from build123d import *

# Parameters (mm, degrees)
SKETCH1_W           = 18.5
SKETCH1_H           = 6
SKETCH1_R           = 1.6
BOSS_EXTRUDE1_DEPTH = 3
SKETCH2_W           = 3
SKETCH2_H           = 6
BOSS_EXTRUDE2_DEPTH = 15.5
SKETCH3_R           = 1.6
CUT_EXTRUDE1_DEPTH  = 25.320773014
BOSS_EXTRUDE3_DEPTH = 6


with BuildPart() as part:
    # Sketch1 → Boss-Extrude1 (new body)
    with BuildSketch(Plane(origin=(0, 0, 0), x_dir=(1, 0, 0), z_dir=(0, 1, 0))):
        Rectangle(SKETCH1_W, SKETCH1_H)
        with Locations(Location((-6.25, 0, 0), (0, 0, 270))):
            Circle(SKETCH1_R, mode=Mode.SUBTRACT)
        with Locations(Location((1.75, 0, 0), (0, 0, 270))):
            Circle(SKETCH1_R, mode=Mode.SUBTRACT)
    extrude(amount=BOSS_EXTRUDE1_DEPTH)

    # Sketch2 → Boss-Extrude2 (add)
    with BuildSketch(Plane(origin=(0, 3, 0), x_dir=(1, 0, 0), z_dir=(0, 1, 0))):
        with Locations((7.75, 0)):
            Rectangle(SKETCH2_W, SKETCH2_H)
    extrude(amount=BOSS_EXTRUDE2_DEPTH)

    # Sketch3 → Cut-Extrude1 (cut, through all)
    with BuildSketch(Plane.ZY.offset(-6.25)):
        with Locations((0, 7)):
            Circle(SKETCH3_R)
        with Locations((0, 15)):
            Circle(SKETCH3_R)
    extrude(amount=-CUT_EXTRUDE1_DEPTH, mode=Mode.SUBTRACT)

    # Sketch5 → Boss-Extrude3 (add)
    with BuildSketch(Plane(origin=(6.25, 3, 3), x_dir=(1, 0, 0), z_dir=(0, 0, 1))):
        Polygon((-1, 0), (0, 1), (0, 0), align=None)
    extrude(amount=-BOSS_EXTRUDE3_DEPTH)


solid = part.part
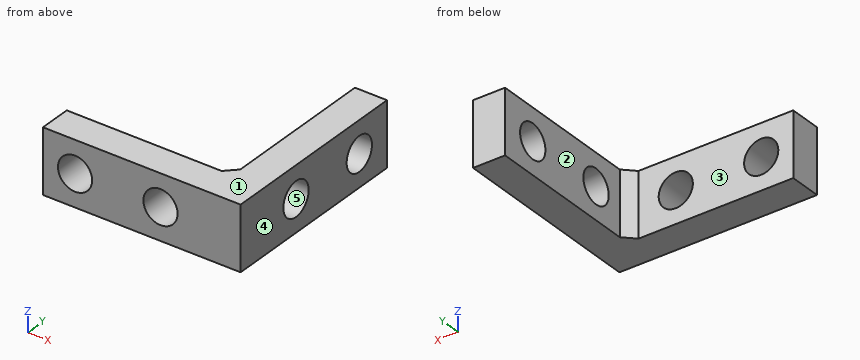
Geometry check sheet. Reference: the model listing, model coordinates, mm. Face numbers are marked on the shaded views. A direction names the side the tool comes from. Give positions to 0.01 mm unless a question says otherwise; leave off trailing zeros. Write each loop counter-clockwise with the first axis right and the second up, starting at its lowest first coordinate (ties: lowest second). Pieces come first, ordered by that corner, then holes. Notation, with made-up numbers: M -8,68.5 L 3,68.5 A23 ccw 3,83.5 Z; hole C 79,-7 d1. An arc over 180 degrees is marked long. Answer as CSV lines item,"result". Start each with the question number.
Q1. Material ranges on L1, parallel to X at y = 1.85, z = 0; L2, parallel to X at y = 12, z = 2.6; L3, parallel to Y at x = 0.5, z = 1.6, recorded low to high.
Q2. Section check B-B, the plane z = 0. Record the cut outline in (x, y), then the cut area to 3 significant figures.
Q3. Section check C-C, the plane y = 7. Record the cut outline in (x, z).
Q4. Section check A-A, the plane x = -6.25. Record the cut outline in (y, z).
Q5. Section check D-D, the plane z = -2.15. Record the cut outline in (x, y), then the cut area to 4 significant figures.
Q6. Go/stop test with flat-tipped pins: pin 1 (3 mm diameter, centred on y = 7, z = 0, fed in from -X); pin 2 (1.5 mm diameter, centred on y = 5.5, z = 2, fed in from -X). Record where each tip stops, or that it passes through.
Q7. Release check for a two-part mould opening along Y. For the marked faces 3, 4 and 5 record: pulls with the +Y half, pulls with the -Y half, needs draft (parallel to the pull), parting line crosses it, or undercut.
Q8. Tool access check on the marked faces 1 and 2. Record the directions out of +Z, -Z, +X, -X, +Y, -Y that give a thin tool (end or side, any length) a straight path to the whole face; none if there is none.
Geometry says:
1,L1,"-9.25 to -7.85, -4.65 to 0.15, 3.35 to 9.25"
1,L2,"6.25 to 9.25"
1,L3,"0 to 3"
2,outline,"M -9.25,0 L -7.85,0 L -7.85,3 L -9.25,3 Z; M -4.65,0 L 0.15,0 L 0.15,3 L -4.65,3 Z; M 3.35,0 L 9.25,0 L 9.25,5.4 L 6.25,5.4 L 6.25,4 L 5.25,3 L 3.35,3 Z; M 6.25,8.6 L 9.25,8.6 L 9.25,13.4 L 6.25,13.4 Z; M 6.25,16.6 L 9.25,16.6 L 9.25,18.5 L 6.25,18.5 Z"
2,area,"64.1 mm^2"
3,outline,"M 6.25,-3 L 9.25,-3 L 9.25,-1.6 L 6.25,-1.6 Z; M 6.25,1.6 L 9.25,1.6 L 9.25,3 L 6.25,3 Z"
4,outline,"M 0,-3 L 3,-3 L 3,-1.6 L 0,-1.6 Z; M 0,1.6 L 3,1.6 L 3,3 L 0,3 Z"
5,outline,"M -9.25,0 L 9.25,0 L 9.25,18.5 L 6.25,18.5 L 6.25,4 L 5.25,3 L -9.25,3 Z"
5,area,"102.5 mm^2"
6,pin 1,"through"
6,pin 2,"x = 6.25"
7,face 3,"pulls with the +Y half"
7,face 4,"needs draft"
7,face 5,"undercut"
8,face 1,"+Z, +X, -X, +Y, -Y"
8,face 2,"+Z, -Z, -X, +Y"
